The model under review builds one solid part; all positions refer to its coordinate system, in mm. A direction names the side the tool comes from. Round coordinates to 2 decimals unless told otherwise and drop trailing zeros. Order: outer loops, then holes, each group sorted by start corner. A loop starts at its lowest first (then second) coordinate and runs counter-clockwise, first axis right, second up. Notation, with made-up numbers: (48.25, 75.25) -> (70.25, 75.25) arc R22 ccw to (70.25, 98.25) -> close; hole circle Ø2 at (10, 59). An arc over 180 degrees is marked (long way). Use a Markdown table: item, result. Add a question column.
```python
from build123d import *

# Parameters (mm, degrees)
SKETCH_1_W          = 4.8
SKETCH_1_H          = 7
EXTRUDE_1_DEPTH     = 15
SKETCH_2_W          = 5
SKETCH_2_H          = 7
EXTRUDE_2_DEPTH     = 5
SKETCH_3_R          = 1.5
CUT_EXTRUDE_1_DEPTH = 15
SKETCH_5_W          = 12
SKETCH_5_H          = 8.8
EXTRUDE_4_DEPTH     = 29.64
CUT_EXTRUDE_2_DEPTH = 2.5
CUT_EXTRUDE_3_REACH = 13
SKETCH_8_R          = 1.5
SKETCH_9_W          = 8.8
SKETCH_9_H          = 8.8
EXTRUDE_5_DEPTH     = 2
CUT_EXTRUDE_5_DEPTH = 2.5
SKETCH_11_R         = 1.5
CUT_EXTRUDE_7_DEPTH = 3.7
SKETCH_12_W         = 4.8
SKETCH_12_H         = 7
CUT_EXTRUDE_8_DEPTH = 10


with BuildPart() as part:
    # 草图1 → 凸台-拉伸1 (new body)
    with BuildSketch(Plane.XY):
        Polygon((-6.8, -0.219543147), (0, -0.219543147), (0, -11.219543147), (-6.8, -11.219543147), (-8.8, -11.219543147), (-8.8, -0.219543147), align=None)
        with Locations((-4.4, -4.719543147)):
            Rectangle(SKETCH_1_W, SKETCH_1_H, mode=Mode.SUBTRACT)
    extrude(amount=EXTRUDE_1_DEPTH)

    # 草图2 → 凸台-拉伸2 (add)
    with BuildSketch(Plane.ZY.offset(2)):
        with Locations((12.5, -4.719543147)):
            Rectangle(SKETCH_2_W, SKETCH_2_H)
    extrude(amount=EXTRUDE_2_DEPTH)

    # 草图3 → 切除-拉伸1 (cut)
    with BuildSketch(Plane.XY.offset(15)):
        with Locations((-4.4, -4.719543147)):
            Circle(SKETCH_3_R)
    extrude(amount=-CUT_EXTRUDE_1_DEPTH, mode=Mode.SUBTRACT)

    # 草图5 → 凸台-拉伸4 (add)
    with BuildSketch(Plane.ZY.offset(8.8)):
        with Locations((9, -7.619543147)):
            Rectangle(SKETCH_5_W, SKETCH_5_H)
    extrude(amount=-EXTRUDE_4_DEPTH)

    # 草图7 → 切除-拉伸2 (cut)
    with BuildSketch(Plane.XY.offset(15)):
        Polygon((-1.195706006, -4.719543147), (-2.797853003, -1.944543147), (-6.002146997, -1.944543147), (-7.604293994, -4.719543147), (-6.002146997, -7.494543147), (-2.797853003, -7.494543147), align=None)
    extrude(amount=-CUT_EXTRUDE_2_DEPTH, mode=Mode.SUBTRACT)

    # 草图8 → 切除-拉伸3 (cut, up to next)
    with BuildSketch(Plane(origin=(0, -11.219543147, 0), x_dir=(-1, 0, 0), z_dir=(0, 1, 0)), mode=Mode.PRIVATE) as cut_extrude_3_sk1:
        with Locations((4.4, 5)):
            Circle(SKETCH_8_R)
    cut_extrude_3_tool1 = extrude(cut_extrude_3_sk1.sketch, amount=CUT_EXTRUDE_3_REACH, mode=Mode.PRIVATE) & part.part
    add(cut_extrude_3_tool1.solids().sort_by_distance((-4.4, -11.219543, 5))[0], mode=Mode.SUBTRACT)

    # 草图9 → 凸台-拉伸5 (add)
    with BuildSketch(Plane(origin=(0, -11.219543147, 0), x_dir=(-1, 0, 0), z_dir=(0, 1, 0))):
        with Locations((4.4, 5)):
            Rectangle(SKETCH_9_W, SKETCH_9_H)
    extrude(amount=-EXTRUDE_5_DEPTH)

    # 草图10 → 切除-拉伸5 (cut)
    with BuildSketch(Plane.XZ.offset(13.219543147)):
        Polygon((-4.4, 1.795706006), (-1.625, 3.397853003), (-1.625, 6.602146997), (-4.4, 8.204293994), (-7.175, 6.602146997), (-7.175, 3.397853003), align=None)
    extrude(amount=-CUT_EXTRUDE_5_DEPTH, mode=Mode.SUBTRACT)

    # 草图11 → 切除-拉伸7 (cut)
    with BuildSketch(Plane(origin=(0, -3.219543147, 0), x_dir=(-1, 0, 0), z_dir=(0, 1, 0))):
        with Locations((-11.84, 8)):
            Circle(SKETCH_11_R)
    extrude(amount=-CUT_EXTRUDE_7_DEPTH, mode=Mode.SUBTRACT)

    # 草图12 → 切除-拉伸8 (cut)
    with BuildSketch(Plane(origin=(0, 0, 0), x_dir=(-1, 0, 0), z_dir=(0, 0, -1))):
        with Locations((4.4, -4.719543147)):
            Rectangle(SKETCH_12_W, SKETCH_12_H)
    extrude(amount=-CUT_EXTRUDE_8_DEPTH, mode=Mode.SUBTRACT)


solid = part.part
```
Q1. Insertion check: pin 1 (0.6 mm diameter, centred on x = -4.5, y = -12, fed in from -Z); pin 2 (3.5 mm diameter, centred on x = 12.5, z = 9, fed in from +Y); pin 3 (2 mm diameter, centred on x = -3.5, z = 13.5, fed in from -Y). Each pin has a flat end and moves straight along its axis. Give the tip position at first contact, or say it passes through.
Q2. Machinability: for faces 1 (the flat face through (10, -8, 3)), 2 (the flat face through (-7.175, -12, 5)), 3 (the cylindrical face through (13.03, -5.04, 7.09)), 4 (the flat face through (-6, -8.22, 4)), which of the approach directions +Z, -Z, +X, -X, +Y, -Y give a long, thin tool a straight path to every point of the face, cutting with its end or side? Answer none if there is none.
Q3. Add section C-C (z = 7). Write out the cut boundary in (x, y), then the cut area to 3 significant figures.
Q4. Add section D-D (x = 16.5). Write out the cut boundary in (y, z).
Q5. Add section A-A (z = 5). Write out the cut boundary in (x, y) (3 decimals), then the cut area to 3 significant figures.
Q6. Mouldability with a two-part tool opening along Y and no side actions: class faces 5 (the flat face through (-4, -12, 0.6)), 6 (the flat face through (-4, -0.22, 7)), 7 (the flat face through (-6.79, -3.31, 13.77)) as pulls with the +Y half, pulls with the -Y half, needs draft (parallel to the pull), parting line crosses it, or undercut.
Q7. Add section B-B (x = 11.84). Write out the cut boundary in (y, z), then the cut area to 3 significant figures.
Q8. Wall thickness on line 1 (X direction, y = -1.5, z = 3); line 2 (Z direction, x = 11.84, y = -5.2); line 3 (X direction, y = -3.5, z = 8.75): over which ranges is each line inside the solid? List them lowest first. Write a range as [from, to].
Report:
| question | item | result |
|---|---|---|
| 1 | pin 1 | stops at z = 0.6 |
| 1 | pin 2 | stops at y = -3.22 |
| 1 | pin 3 | stops at y = -12.02 |
| 2 | face 1 | -Z, +X, +Y, -Y |
| 2 | face 2 | -Y |
| 2 | face 3 | +Y |
| 2 | face 4 | -Z |
| 3 | outline | (-8.8, -13.22) -> (-6.49, -13.22) -> (-6.49, -10.72) -> (-2.31, -10.72) -> (-2.31, -13.22) -> (0, -13.22) -> (0, -12.02) -> (20.84, -12.02) -> (20.84, -3.22) -> (12.96, -3.22) -> (12.96, -6.92) -> (10.72, -6.92) -> (10.72, -3.22) -> (0, -3.22) -> (0, -0.22) -> (-8.8, -0.22) -> close; hole (-6.8, -8.22) -> (-2, -8.22) -> (-2, -1.22) -> (-6.8, -1.22) -> close |
| 3 | area | 245 mm² |
| 4 | outline | (-12.02, 3) -> (-3.22, 3) -> (-3.22, 15) -> (-12.02, 15) -> close |
| 5 | outline | (-8.8, -13.22) -> (-7.175, -13.22) -> (-7.175, -10.72) -> (-5.9, -10.72) -> (-5.9, -8.22) -> (-6.8, -8.22) -> (-6.8, -1.22) -> (-2, -1.22) -> (-2, -8.22) -> (-2.9, -8.22) -> (-2.9, -10.72) -> (-1.625, -10.72) -> (-1.625, -13.22) -> (0, -13.22) -> (0, -12.02) -> (20.84, -12.02) -> (20.84, -3.22) -> (0, -3.22) -> (0, -0.22) -> (-8.8, -0.22) -> close |
| 5 | area | 243 mm² |
| 6 | face 5 | needs draft |
| 6 | face 6 | pulls with the +Y half |
| 6 | face 7 | undercut |
| 7 | outline | (-12.02, 3) -> (-3.22, 3) -> (-3.22, 6.5) -> (-6.92, 6.5) -> (-6.92, 9.5) -> (-3.22, 9.5) -> (-3.22, 15) -> (-12.02, 15) -> close |
| 7 | area | 94.5 mm² |
| 8 | line 1 | x = [-8.8, -6.8], [-2, 0] |
| 8 | line 2 | z = [3, 6.5], [9.5, 15] |
| 8 | line 3 | x = [-8.8, -6.8], [-2, 10.54], [13.14, 20.84] |
